from build123d import *

# Parameters (mm, degrees)
SKETCH1_W          = 254
SKETCH1_H          = 3.175
BASE_FLANGE1_DEPTH = 76.2
SKETCH6_R          = 12.7
CUT_EXTRUDE1_DEPTH = 266.202791511
SKETCH7_R          = 2.286
CUT_EXTRUDE2_DEPTH = 266.202791511
SKETCH8_R          = 2.286
CUT_EXTRUDE3_DEPTH = 266.202791511
SKETCH9_R          = 3.556
CUT_EXTRUDE4_DEPTH = 266.202791511


# Sheet-metal steps are written as plain solids
with BuildPart() as part:
    # Sketch1 → Base-Flange1 (new, symmetric)
    with BuildSketch(Plane.XY):
        with Locations((-127, 1.5875)):
            Rectangle(SKETCH1_W, SKETCH1_H)
    extrude(amount=BASE_FLANGE1_DEPTH, both=True)

    # Sketch6 → Cut-Extrude1 (cut, through all)
    with BuildSketch(Plane.XZ):
        with Locations(Location((-140.208, 0, 0), (0, 0, 270))):
            Circle(SKETCH6_R)
    extrude(amount=-CUT_EXTRUDE1_DEPTH, mode=Mode.SUBTRACT)

    # Sketch7 → Cut-Extrude2 (cut, through all)
    with BuildSketch(Plane.XZ):
        with Locations(Location((-107.188, 0, 0), (0, 0, 270))):
            Circle(SKETCH7_R)
        with Locations(Location((-173.228, 0, 0), (0, 0, 90))):
            Circle(SKETCH7_R)
    extrude(amount=-CUT_EXTRUDE2_DEPTH, mode=Mode.SUBTRACT)

    # Sketch8 → Cut-Extrude3 (cut, through all)
    with BuildSketch(Plane.XZ):
        with Locations(Location((-140.208, -37.338, 0), (0, 0, 90))):
            Circle(SKETCH8_R)
    extrude(amount=-CUT_EXTRUDE3_DEPTH, mode=Mode.SUBTRACT)

    # Sketch9 → Cut-Extrude4 (cut, through all)
    with BuildSketch(Plane(origin=(0, 3.175, 0), x_dir=(1, 0, 0), z_dir=(0, 1, 0))):
        with Locations(Location((-173.228, 53.34, 0), (0, 0, 270))):
            Circle(SKETCH9_R)
        with Locations(Location((-80.772, 53.34, 0), (0, 0, 90))):
            Circle(SKETCH9_R)
    extrude(amount=-CUT_EXTRUDE4_DEPTH, mode=Mode.SUBTRACT)


solid = part.part
Check sheet for the modelled part. Datum: model origin and axes. Units: mm. Round coordinates to 2 decimals unless told otherwise and drop trailing zeros. Loops run counter-clockwise (first coordinate to the right, second up) from the corner with the lowest first, then second, coordinate; pieces in that order, holes last. Notation, with made-up numbers: M -35.5,4.25 L 4.5,4.25 A8 cw 4.5,11.25 Z; hole C 56.25,66 d2. An arc over 180 degrees is marked long. One line per item, written item: value.
(1) Sectioned sample at C-C, the plane y = 0.5. Record the cut outline in (x, z), then the cut area to 3 significant figures.
Computed values:
outline: M -254,-76.2 L 0,-76.2 L 0,76.2 L -254,76.2 Z; hole C -173.23,-53.34 d7.11; hole C -173.23,0 d4.57; hole C -140.21,0 d25.4; hole C -140.21,-37.34 d4.57; hole C -107.19,0 d4.57; hole C -80.77,-53.34 d7.11
area: 38,100 mm^2
(2) Thickness scan on line 1 (X direction, y = 1.2, z = 0); line 2 (Z direction, x = -148, y = 1.3); line 3 (Z direction, x = -77.5, y = 2.5). Record the ranges inside material, lowest first.
Computed values:
line 1: x = -254 to -175.51, -170.94 to -152.91, -127.51 to -109.47, -104.9 to 0
line 2: z = -76.2 to -10.03, 10.03 to 76.2
line 3: z = -76.2 to -54.73, -51.95 to 76.2
(3) Sectioned sample at D-D, the plane z = -9.5. Record the cut outline in (x, y) (3 decimals), then the cut area to 3 significant figures.
Computed values:
outline: M -254,0 L -148.637,0 L -148.637,3.175 L -254,3.175 Z; M -131.779,0 L 0,0 L 0,3.175 L -131.779,3.175 Z
area: 753 mm^2
(4) Sectioned sample at B-B, the plane x = -146. Record the cut outline in (y, z) (3 decimals).
Computed values:
outline: M 0,-76.2 L 3.175,-76.2 L 3.175,-11.302 L 0,-11.302 Z; M 0,11.302 L 3.175,11.302 L 3.175,76.2 L 0,76.2 Z
(5) Release check for a two-part mould opening along Z. For faces 1 (the face through (-129, 3.175, 18)), 2 (the face through (-83.175, 1.61, -50.719)) record: +Z half, -Z half, draft (parallel to the pull), parting line (faces both ways), or undercut.
Computed values:
face 1: draft
face 2: undercut
(6) Sectioned sample at A-A, the plane z = -53.34. Record the cut outline in (x, y) (3 decimals).
Computed values:
outline: M -254,0 L -176.784,0 L -176.784,3.175 L -254,3.175 Z; M -169.672,0 L -84.328,0 L -84.328,3.175 L -169.672,3.175 Z; M -77.216,0 L 0,0 L 0,3.175 L -77.216,3.175 Z
